For this review, use the dimensioned drawing (mm, ordinates from the lowest corner) and the shaded views. A direction names the side the tool comes from. Round coordinates to 2 decimals unless told otherwise and drop trailing zeros. Order: outer loops, then holes, each group sorted by start corner. A loop starts at its lowest first (then second) coordinate and runs counter-clockwise, first axis right, second up. Notation, with made-up numbers: (-39, 41) - (-11, 41) arc R23 cw to (-11, 53) - close; hole circle Ø5 at (-9, 56). An arc over 180 degrees is marked (long way). Use CSV: the item, a comma, the result in double quotes. Start each with the question number.
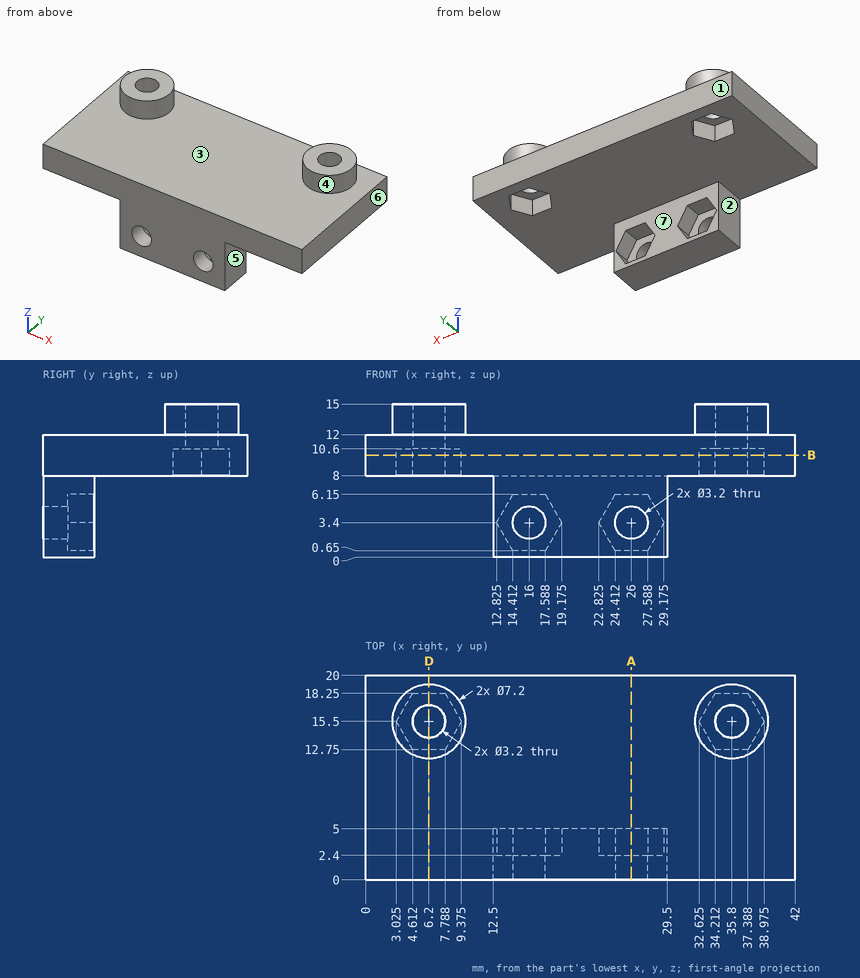
Q1. Take a section at D-D (x = 6.2). State the section outline as (y, z) points.
Q2. For L1, parallel to Z at x = 26, y = 0.6; L2, parallel to Y at x = 35.8, z = 13.95; L3, parallel to Y at x = 36, z = 9, list the stretches that pass through material, from the lowest coordinate up. Write a range as [from, to].
Q3. Clearance check with flat-ended pins moving along their axes: pin 1 (10 mm diameter, centred on x = 23.5, y = 4, fed in from +Z); pin 2 (4 mm diameter, centred on y = 8, z = 11.5, fed in from -X); pin 3 (4.5 mm diameter, centred on x = 24.5, z = 3, fed in from +Y); pin 4 (4 mm diameter, centred on y = 2, z = 5.5, fed in from -X). State where each tip first meets the part, or that it passes through.
Q4. Tool access review of the marked faces 4, 5, 6 and 7: name each direction out of +Z, -Z, +X, -X, +Y, -Y from which nothing blocks a thin tool from reaching the whole face with its end or side.
Q5. Take a section at A-A (x = 26). State the section outline as (y, z) points.
Q6. The part is to be moulded in two halves that separate along X. For the marked faces 1, 2 and 3, say which applies: +X half, -X half, draft (parallel to the pull), parting line (faces both ways), or undercut.
Q7. Take a section at B-B (z = 10). Give the number of separate pieces and of enclosed holes in the cut face.
Findings below:
1,outline,"(0, 8) - (12.75, 8) - (12.75, 10.6) - (13.9, 10.6) - (13.9, 15) - (11.9, 15) - (11.9, 12) - (0, 12) - close; (17.1, 10.6) - (18.25, 10.6) - (18.25, 8) - (20, 8) - (20, 12) - (19.1, 12) - (19.1, 15) - (17.1, 15) - close"
2,L1,"z = [0, 1.8], [5, 12]"
2,L2,"y = [11.9, 13.9], [17.1, 19.1]"
2,L3,"y = [0, 12.75], [18.25, 20]"
3,pin 1,"stops at z = 12"
3,pin 2,"stops at x = 0"
3,pin 3,"stops at y = 5"
3,pin 4,"stops at x = 12.5"
4,face 4,"+Z"
4,face 5,"-Z, +X, +Y, -Y"
4,face 6,"+Z, -Z, +X, +Y, -Y"
4,face 7,"-Z, +X, -X, +Y"
5,outline,"(0, 0) - (5, 0) - (5, 0.65) - (2.4, 0.65) - (2.4, 1.8) - (0, 1.8) - close; (0, 5) - (2.4, 5) - (2.4, 6.15) - (5, 6.15) - (5, 8) - (20, 8) - (20, 12) - (0, 12) - close"
6,face 1,"draft"
6,face 2,"-X half"
6,face 3,"undercut"
7,separate pieces,"1"
7,enclosed holes,"2"
